Could you check a few things on this model? Use its own coordinates, in mm. A direction names the side the tool comes from. Round coordinates to 2 decimals unless told otherwise and drop trailing zeros. Loops run counter-clockwise (first coordinate to the right, second up) from the corner with the lowest first, then second, coordinate; pieces in that order, holes last. Notation, with made-up numbers: (82.25, -7.75) -> (94.25, -7.75) arc R15 cw to (94.25, 16.25) -> close; hole circle Ø9 at (-12, -25.75). An arc over 180 degrees is marked (long way). One line per item, written item: value.
```python
from build123d import *

# Parameters (mm, degrees)
SKETCH1_R           = 10
BOSS_EXTRUDE1_DEPTH = 15
CUT_EXTRUDE1_DEPTH  = 16
CUT_EXTRUDE2_DEPTH  = 10
CUT_EXTRUDE3_DEPTH  = 10


with BuildPart() as part:
    # Sketch1 → Boss-Extrude1 (new body)
    with BuildSketch(Plane.XY):
        Circle(SKETCH1_R)
    extrude(amount=BOSS_EXTRUDE1_DEPTH)

    # Sketch2 → Cut-Extrude1 (cut, through all)
    with BuildSketch(Plane.XY.offset(15)):
        with BuildLine():
            Line((0, 0), (10, 0))
            ThreePointArc((10, 0), (7.071067812, -7.071067812), (0, -10))
            Line((0, -10), (0, 0))
        make_face()
    extrude(amount=-CUT_EXTRUDE1_DEPTH, mode=Mode.SUBTRACT)

    # Sketch5 → Cut-Extrude2 (cut)
    with BuildSketch(Plane(origin=(10, 0, 0), x_dir=(0, 0, -1), z_dir=(1, 0, 0))):
        Polygon((0, 0), (0, 10), (-15, 10), align=None)
    extrude(amount=-CUT_EXTRUDE2_DEPTH, mode=Mode.SUBTRACT)

    # Sketch6 → Cut-Extrude3 (cut)
    with BuildSketch(Plane(origin=(0, 0, 0), x_dir=(0, 0, -1), z_dir=(1, 0, 0))):
        Polygon((-15, 10), (0, 0), (0, 10), align=None)
    extrude(amount=-CUT_EXTRUDE3_DEPTH, mode=Mode.SUBTRACT)


solid = part.part
```
(1) For pin 1 Ø3 at (y, z) = (-0.5, 8) entering from -X; pin 2 Ø2 at (y, z) = (-4, 2) entering from +X; pin 3 Ø5 at (x, z) = (5, 9) entering from -Y; pin 4 Ø1 at (x, z) = (-6.5, 9) entering from +Y, each with a flat end and sliding along its axis, tell me the tip position at first contact or that it passes through.
Results below:
pin 1: stops at x = -10
pin 2: stops at x = 0
pin 3: stops at y = 0
pin 4: stops at y = 6.33
(2) Imagine slicing it at C-C on y = 8. Write out the boundary of the cut face in (x, z), then the cut area to 3 significant figures.
Results below:
outline: (-6, 12) -> (6, 12) -> (6, 15) -> (-6, 15) -> close
area: 36.0 mm²
(3) On a 3-axis mill with a long thin cutter (end or side, diameter ignored), from which of +Z, -Z, +X, -X, +Y, -Y can I reach the whole of each face in a straight line? I mean faces 1 (the face through (0, -5, 8)), 2 (the face through (-4, -4, 0)). Say none if no direction works.
Results below:
face 1: +Z, -Z, +X, -Y
face 2: -Z, +X, -X, +Y, -Y
(4) Please list where these lines run through material, in increasing order: L1, parallel to X at y = -1.5, z = 5.5; L2, parallel to X at y = 3.5, z = 7; L3, parallel to Z at x = -5.25, y = 1.5.
Results below:
L1: x = -9.89 to 0
L2: x = -9.37 to 9.37
L3: z = 2.25 to 15
(5) Imagine slicing it at A-A on z = 10.75. Write out the boundary of the cut face in (x, y).
Results below:
outline: (-6.97, 7.17) arc R10 ccw to (0, -10) -> (0, 0) -> (10, 0) arc R10 ccw to (6.97, 7.17) -> close
(6) Imagine slicing it at D-D on y = 2.75. Write out the boundary of the cut face in (x, z) (3 decimals), then the cut area to 3 significant figures.
Results below:
outline: (-9.614, 4.125) -> (9.614, 4.125) -> (9.614, 15) -> (-9.614, 15) -> close
area: 209 mm²
(7) Imagine slicing it at B-B on x = -2.5. Write out the boundary of the cut face in (y, z), then the cut area to 3 significant figures.
Results below:
outline: (-9.68, 0) -> (0, 0) -> (9.68, 14.52) -> (9.68, 15) -> (-9.68, 15) -> close
area: 220 mm²
